Geometry check sheet. Reference: drawing and pictorial views, mm from the part's lowest x, y, z. Coordinates: 2 decimals unless noted, no trailing zeros. Write each loop counter-clockwise with the first axis right and the second up, starting at its lowest first coordinate (ties: lowest second). Pieces come first, ordered by that corner, then holes. Notation, with made-up numbers: (1, -32.75) - (55, -32.75) arc R13 ccw to (55, -15.75) - close; hole circle Ø6 at (-9, 50). An arc over 180 degrees is marked (long way). Answer as a JSON object with one key per item and string values. Group by question number.
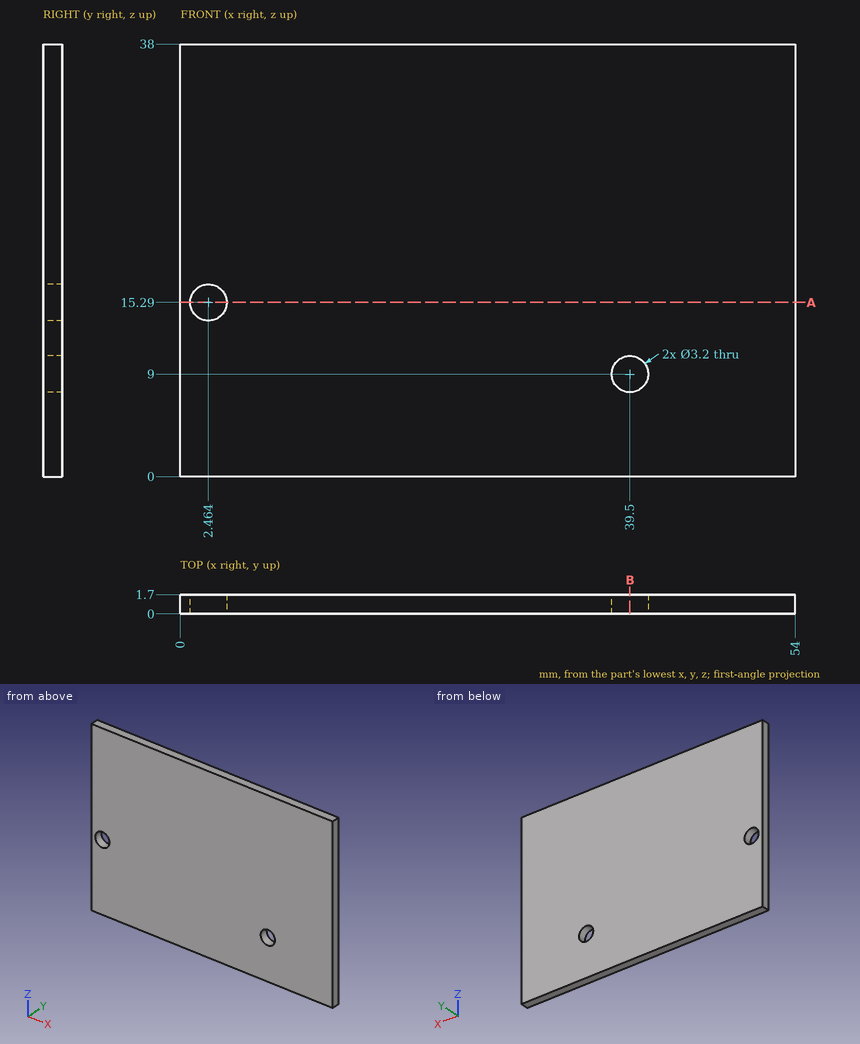
(1) Material ranges on L1, parallel to Z at x = 39.5, y = 1.2; L2, parallel to Z at x = 3, y = 1.2; L3, parallel to X at y = 1.4, z = 15, recorded low to high. Write a range as [from, to].
(2) Section check B-B (x = 39.5). Record the cut outline in (y, z).
(3) Gauge pin test, flat end, axial feed: pin 1 (1.9 mm diameter, centred on x = 39.5, z = 9, fed in from -Y). Record the tip position at first contact, or that the pin passes through.
(4) Section check A-A (z = 15.29). Record the cut outline in (x, y).
Conclusion:
{
 "1": {"L1": "z = [0, 7.4], [10.6, 38]", "L2": "z = [0, 13.78], [16.8, 38]", "L3": "x = [0, 0.89], [4.04, 54]"},
 "2": {"outline": "(0, 0) - (1.7, 0) - (1.7, 7.4) - (0, 7.4) - close; (0, 10.6) - (1.7, 10.6) - (1.7, 38) - (0, 38) - close"},
 "3": {"pin 1": "passes through"},
 "4": {"outline": "(0, 0) - (0.86, 0) - (0.86, 1.7) - (0, 1.7) - close; (4.06, 0) - (54, 0) - (54, 1.7) - (4.06, 1.7) - close"}
}
